```python
from build123d import *

# Parameters (mm, degrees)
F0_W          = 914.4
F0_H          = 914.4
F1_DEPTH      = 914.4
F2_W          = 243.84
F2_H          = 243.84
F3_DEPTH      = 335.28
F4_W          = 243.84
F4_H          = 243.84
F5_DEPTH      = 812.9016
F6_W          = 188.6856555939
F6_H          = 60.96
F6_W_2        = 60.96
F6_H_2        = 188.6712
F7_DEPTH      = 50.81016
F7_DEPTH_BACK = 30.48


# Not quite as in the source:
# - a feature names something its author has since deleted; it is built from what else it names


with BuildPart() as f1:
    # F0 (on Front) → F1 (new body)
    with BuildSketch(Plane.XZ):
        Rectangle(F0_W, F0_H)
    extrude(amount=F1_DEPTH)

    # F2 (on face) → F3 (cut)
    with BuildSketch(Plane.XZ.offset(914.4)):
        with Locations((0, -233.7816)):
            Rectangle(F2_W, F2_H)
    extrude(amount=-F3_DEPTH, mode=Mode.SUBTRACT)

    # F4 (on face) → F5 (cut)
    with BuildSketch(Plane.XY.offset(457.2)):
        with Locations((0, -457.2)):
            Rectangle(F4_W, F4_H)
    extrude(amount=-F5_DEPTH, mode=Mode.SUBTRACT)

    # F6 (on face) → F7 (join, two sides)
    with BuildSketch(Plane.XY.offset(457.2)) as f7_sk:
        with Locations((240.9371722031, -457.2)):
            Rectangle(F6_W, F6_H)
        with Locations((0, -216.2556)):
            Rectangle(F6_W_2, F6_H_2)
        with Locations((-240.9371722031, -457.2)):
            Rectangle(F6_W, F6_H)
        with Locations((0, -698.1444)):
            Rectangle(F6_W_2, F6_H_2)
    extrude(amount=F7_DEPTH)
    extrude(f7_sk.sketch, amount=-F7_DEPTH_BACK)


solid = f1.part
```
Could you check a few things on this model? Use its own coordinates, in mm. A direction names the side the tool comes from. Round coordinates to 2 decimals unless told otherwise and drop trailing zeros. Order: outer loops, then holes, each group sorted by start corner. A loop starts at its lowest first (then second) coordinate and runs counter-clockwise, first axis right, second up. Notation, with made-up numbers: M 28.25,69.25 L 79.25,69.25 A18 cw 79.25,87.25 Z; hole C -31.5,68.5 d5. An arc over 180 degrees is marked long. One line per question, with ' | ' between items. Start each with the question number.
(1) Thinking about a two-plate mould opening in X: for faces 4 (the face through (-146.594, -458, 482)), 5 (the face through (30.48, -699, 482)), 6 (the face through (0, -697, 508.01)), 7 (the face through (-335.28, -458, 482)), which applies, +X half, -X half, draft (parallel to the pull), parting line (faces both ways), or undercut?
(2) Suppose I cut it at A-A on x = 14.5. List the corners of the cut face in (y, z) for me.
(3) Please list where these lines run through material, in increasing order: line 1 along X through (y, z) = (-555, -348); line 2 along Z through (x, y) = (-100, -425.5); line 3 along Z through (x, y) = (-175, -281).
(4) For faces 1 (the face through (-242, -426.72, 482)), 2 (the face through (30.48, -218, 482)), 3 (the face through (-242, -487.68, 482)), which set-ups out of +Z, -Z, +X, -X, +Y, -Y let a thin tool reach every point of the face, with its end or its side?
(5) Suppose I cut it at C-C on z = 111.5. List the corners of the cut face in (x, y) for me.
(6) For P1, Ø15, axis at x = -10, z = 492.5, coming from the -Y side; P2, Ø15, axis at y = -245, z = 473, coming from the -X side; P3, Ø1.5, axis at x = 131.5, y = -473.5, coming from the +Z side, each with a flat end and sliding along its axis, tell me the tip position at first contact or that it passes through.
(7) Suppose I cut it at B-B on y = -650.5. List the corners of the cut face in (x, z) for me, then the cut area to 3 significant figures.
(8) Suppose I cut it at D-D on x = 281. List the corners of the cut face in (y, z) for me, then the cut area to 3 significant figures.
Geometry results:
1) face 4: undercut | face 5: +X half | face 6: draft | face 7: -X half
2) outline: M -914.4,-457.2 L 0,-457.2 L 0,457.2 L -121.92,457.2 L -121.92,508.01 L -310.59,508.01 L -310.59,457.2 L -335.28,457.2 L -335.28,-355.7 L -914.4,-355.7 Z; M -914.4,-111.86 L -579.12,-111.86 L -579.12,457.2 L -603.81,457.2 L -603.81,508.01 L -792.48,508.01 L -792.48,457.2 L -914.4,457.2 Z
3) line 1: -457.2 to -121.92, 121.92 to 457.2 | line 2: -457.2 to -355.7 | line 3: -457.2 to 457.2
4) face 1: +Z, +X, -X, +Y | face 2: +Z, +X, +Y, -Y | face 3: +Z, +X, -X, -Y
5) outline: M -457.2,-914.4 L 457.2,-914.4 L 457.2,0 L -457.2,0 Z; hole M -121.92,-579.12 L 121.92,-579.12 L 121.92,-335.28 L -121.92,-335.28 Z
6) P1: y = -792.48 | P2: x = -30.48 | P3: z = 457.2
7) outline: M -457.2,-457.2 L 457.2,-457.2 L 457.2,457.2 L 30.48,457.2 L 30.48,508.01 L -30.48,508.01 L -30.48,457.2 L -457.2,457.2 Z; hole M -121.92,-355.7 L 121.92,-355.7 L 121.92,-111.86 L -121.92,-111.86 Z | area: 780,000 mm²
8) outline: M -914.4,-457.2 L 0,-457.2 L 0,457.2 L -426.72,457.2 L -426.72,508.01 L -487.68,508.01 L -487.68,457.2 L -914.4,457.2 Z | area: 839,000 mm²
